Check sheet for the modelled part. Datum: model origin and axes. Units: mm. Face numbers are marked on the shaded views. A direction names the side the tool comes from. Round coordinates to 2 decimals unless told otherwise and drop trailing zeros. Loops run counter-clockwise (first coordinate to the right, second up) from the corner with the lowest first, then second, coordinate; pieces in that order, holes last. Notation, with made-up numbers: (69.5, 73.5) - (123.5, 73.5) arc R25 cw to (123.5, 110.5) - close; hole circle Ø2 at (28, 56.25). An arc over 180 degrees is marked (long way). Return JSON: item names as keys, results as strings.
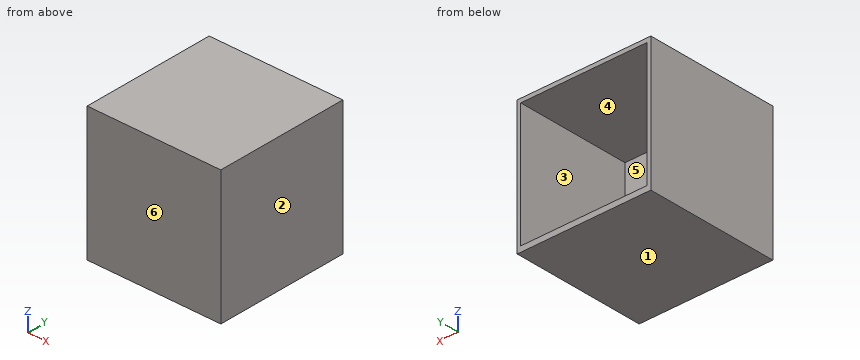
from build123d import *

# Parameters (mm, degrees)
F0_W     = 50.8
F0_H     = 50.8
F1_DEPTH = 50.8
F2_W     = 47.9298
F2_H     = 47.1678
F3_DEPTH = 43.434


with BuildPart() as f1:
    # F0 (on Right) → F1 (new body)
    with BuildSketch(Plane.YZ):
        with Locations((-25.4, 25.4)):
            Rectangle(F0_W, F0_H)
    extrude(amount=F1_DEPTH)

    # F2 (on Front) → F3 (cut)
    with BuildSketch(Plane.XZ):
        with Locations((25.492538, 25.684401)):
            Rectangle(F2_W, F2_H)
    extrude(amount=F3_DEPTH, mode=Mode.SUBTRACT)


solid = f1.part
Q1. Scan lines: probe 1 along Z at (x, y) = (12, -8.5); probe 2 along X at (y, z) = (-31, 34); probe 3 along Y at (x, z) = (25, 3.5). Record each from-to range of solid material in increasing order. Write a range as [from, to].
Answer key:
{"probe 1": "z = [0, 2.1], [49.27, 50.8]", "probe 2": "x = [0, 1.53], [49.46, 50.8]", "probe 3": "y = [-50.8, -43.43]"}
Q2. Sectioned sample at A-A (y = -42). Enter the section's corners in (x, z).
Answer key:
{"outline": "(0, 0) - (50.8, 0) - (50.8, 50.8) - (0, 50.8) - close; hole (1.53, 2.1) - (49.46, 2.1) - (49.46, 49.27) - (1.53, 49.27) - close"}
Q3. Sectioned sample at C-C (x = 8). Enter the section's corners in (y, z).
Answer key:
{"outline": "(-50.8, 0) - (0, 0) - (0, 2.1) - (-43.43, 2.1) - (-43.43, 49.27) - (0, 49.27) - (0, 50.8) - (-50.8, 50.8) - close"}
Q4. Depth check by flat-ended pin: P1, Ø6, axis at x = 44.5, z = 33, coming from the +Y side. Enter the tip coordinate at first touch or a pass-through.
Answer key:
{"P1": "stops at y = -43.43"}
Q5. Sectioned sample at B-B (z = 8). Enter the section's corners in (x, y), plus the area to 3 significant figures.
Answer key:
{"outline": "(0, -50.8) - (50.8, -50.8) - (50.8, 0) - (49.46, 0) - (49.46, -43.43) - (1.53, -43.43) - (1.53, 0) - (0, 0) - close", "area": "499 mm²"}
Q6. Tool access check on the marked faces 5 and 6. Record the directions out of +Z, -Z, +X, -X, +Y, -Y that give a thin tool (end or side, any length) a straight path to the whole face; none if there is none.
Answer key:
{"face 5": "+Y", "face 6": "+Z, -Z, +X, -X, -Y"}
Q7. Draft check along Z on the marked faces 1, 2, 3 and 4. Enter one of: released by +Z, released by -Z, zero draft, split by the parting line, or undercut.
Answer key:
{"face 1": "released by -Z", "face 2": "zero draft", "face 3": "undercut", "face 4": "undercut"}
